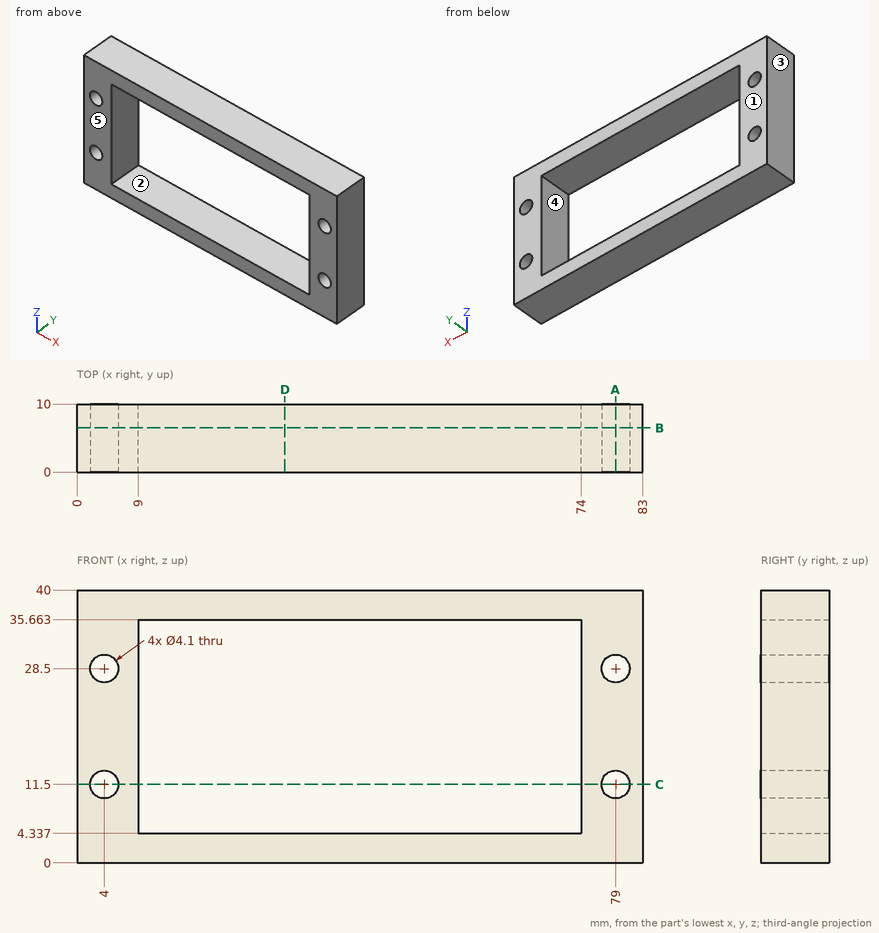
The drawing under review shows one solid part. Ordinate dimensions are in mm from its lowest x, y, z. A direction names the side the tool comes from. Coordinates: 2 decimals unless noted, no trailing zeros. Order: outer loops, then holes, each group sorted by start corner. A loop starts at its lowest first (then second) coordinate and runs counter-clockwise, first axis right, second up. Notation, with made-up numbers: (-27.5, 19) -> (24.5, 19) arc R16 cw to (24.5, 45) -> close; hole circle Ø7 at (60.25, 89.5). An arc over 180 degrees is marked (long way). Answer in a Markdown table with one row per item. Add a question column.
Item 1: To check wall thickness, follow probe 1 along Z at (x, y) = (4, 7.75); probe 2 along X at (y, z) = (4.25, 28.5); probe 3 along Z at (x, y) = (59, 7.25). State the ranges of each line that lie inside material, in increasing order.
Item 2: Machinability: for the marked faces 1 and 2, which of the approach directions +Z, -Z, +X, -X, +Y, -Y give a long, thin tool a straight path to every point of the face, cutting with its end or side? Answer none if there is none.
Item 3: We need section C-C on z = 11.5. Write out the cut boundary in (x, y).
Item 4: Clearance check with a flat-ended pin moving along its axis: pin 1 (1.5 mm diameter, centred on x = 39, y = 8.5, fed in from -Z). State where the tip first meets the part, or that it passes through.
Item 5: Mouldability with a two-part tool opening along X and no side actions: class the marked faces 3, 4 and 5 as +X half, -X half, draft (parallel to the pull), parting line (faces both ways), or undercut.
Item 6: We need section D-D on x = 30.5. Write out the cut boundary in (y, z).
Item 7: We need section A-A on x = 79. Write out the cut boundary in (y, z), plus the area to 3 significant figures.
Item 8: We need section B-B on y = 6.5. Write out the cut boundary in (x, z), plus the area to 3 significant figures.
Final values:
| question | item | result |
|---|---|---|
| 1 | probe 1 | z = 0 to 9.45, 13.55 to 26.45, 30.55 to 40 |
| 1 | probe 2 | x = 0 to 1.95, 6.05 to 9, 74 to 76.95, 81.05 to 83 |
| 1 | probe 3 | z = 0 to 4.34, 35.66 to 40 |
| 2 | face 1 | +Z, -Z, +X, -X, +Y |
| 2 | face 2 | +Y, -Y |
| 3 | outline | (0, 0) -> (1.95, 0) -> (1.95, 10) -> (0, 10) -> close; (6.05, 0) -> (9, 0) -> (9, 10) -> (6.05, 10) -> close; (74, 0) -> (76.95, 0) -> (76.95, 10) -> (74, 10) -> close; (81.05, 0) -> (83, 0) -> (83, 10) -> (81.05, 10) -> close |
| 4 | pin 1 | stops at z = 0 |
| 5 | face 3 | -X half |
| 5 | face 4 | undercut |
| 5 | face 5 | draft |
| 6 | outline | (0, 0) -> (10, 0) -> (10, 4.34) -> (0, 4.34) -> close; (0, 35.66) -> (10, 35.66) -> (10, 40) -> (0, 40) -> close |
| 7 | outline | (0, 0) -> (10, 0) -> (10, 9.45) -> (0, 9.45) -> close; (0, 13.55) -> (10, 13.55) -> (10, 26.45) -> (0, 26.45) -> close; (0, 30.55) -> (10, 30.55) -> (10, 40) -> (0, 40) -> close |
| 7 | area | 318 mm2 |
| 8 | outline | (0, 0) -> (83, 0) -> (83, 40) -> (0, 40) -> close; hole circle Ø4.1 at (4, 11.5); hole circle Ø4.1 at (4, 28.5); hole (9, 4.34) -> (74, 4.34) -> (74, 35.66) -> (9, 35.66) -> close; hole circle Ø4.1 at (79, 11.5); hole circle Ø4.1 at (79, 28.5) |
| 8 | area | 1,230 mm2 |
